Drawing for the job (mm, zero at the part's lowest x, y, z). Give positions to 0.01 mm unless a question says otherwise; leave off trailing zeros. Loops run counter-clockwise (first coordinate to the right, second up) from the corner with the lowest first, then second, coordinate; pieces in that order, holes last. Notation, with made-up numbers: (80, 7.25) -> (129, 7.25) arc R21 cw to (129, 35.25) -> close; hole circle Ø7 at (33, -1.75). An arc over 180 degrees is marked (long way). Answer in a Markdown table with one row per item. Add a question column.
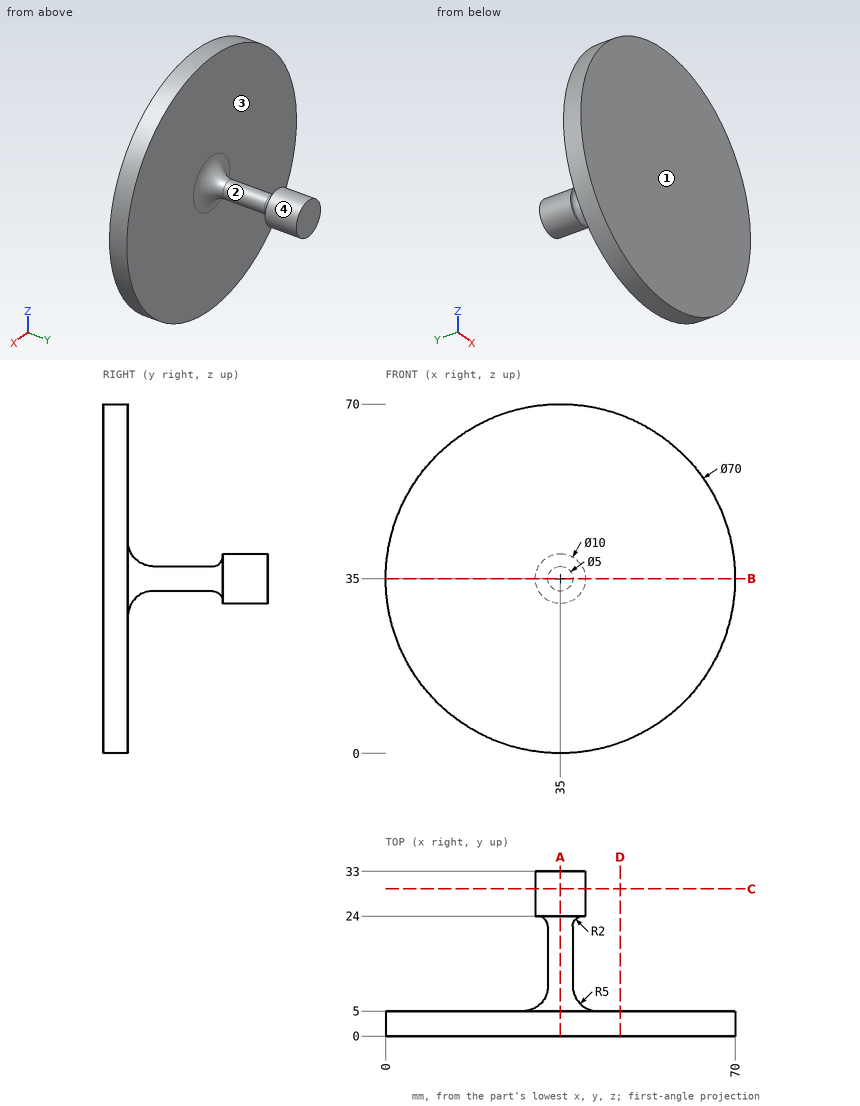
(1) Flat gauge pins, fed straight in: pin 1 Ø5 at (x, z) = (36.5, 33) entering from -Y; pin 2 Ø4 at (x, y) = (27.5, 22) entering from +Z; pin 3 Ø4 at (x, z) = (13.5, 32) entering from +Y; pin 4 Ø10 at (x, y) = (28, 8.5) entering from -Z. Where does each tip first touch, or does it go through?
(2) Wall check: line 1 along Y through (x, z) = (51, 53.5); line 2 along Y through (x, z) = (36, 30); line 3 along X through (y, z) = (3.5, 28). Give the ranges that are in metal, low to high. Write a range as from..to.
(3) Saw through at B-B, the plane z = 35. List the corners of the cut face in (x, y).
(4) Saw through at C-C, the plane y = 29.5. List the corners of the cut face in (x, z).
(5) Two-plate mould, pull along Y, no slides. Class the marked faces 1, 2, 3 and 4: released by +Y, released by -Y, zero draft, split by the parting line, or undercut.
(6) Saw through at D-D, the plane x = 47. List the corners of the cut face in (y, z), then the cut area to 3 significant figures.
(7) Saw through at A-A, the plane x = 35. List the corners of the cut face in (y, z), then the cut area to 3 significant figures.
Worked answers:
| question | item | result |
|---|---|---|
| 1 | pin 1 | y = 0 |
| 1 | pin 2 | through |
| 1 | pin 3 | y = 5 |
| 1 | pin 4 | z = 0.17 |
| 2 | line 1 | 0..5 |
| 2 | line 2 | 0..5.61 |
| 2 | line 3 | 0.71..69.29 |
| 3 | outline | (0, 0) -> (70, 0) -> (70, 5) -> (42.5, 5) arc R5 cw to (37.5, 10) -> (37.5, 22) arc R2 cw to (39.5, 24) -> (40, 24) -> (40, 33) -> (30, 33) -> (30, 24) -> (30.5, 24) arc R2 cw to (32.5, 22) -> (32.5, 10) arc R5 cw to (27.5, 5) -> (0, 5) -> close |
| 4 | outline | circle Ø10 at (35, 35) |
| 5 | face 1 | released by -Y |
| 5 | face 2 | undercut |
| 5 | face 3 | released by +Y |
| 5 | face 4 | zero draft |
| 6 | outline | (0, 2.12) -> (5, 2.12) -> (5, 67.88) -> (0, 67.88) -> close |
| 6 | area | 329 mm^2 |
| 7 | outline | (0, 0) -> (5, 0) -> (5, 27.5) arc R5 cw to (10, 32.5) -> (22, 32.5) arc R2 cw to (24, 30.5) -> (24, 30) -> (33, 30) -> (33, 40) -> (24, 40) -> (24, 39.5) arc R2 cw to (22, 37.5) -> (10, 37.5) arc R5 cw to (5, 42.5) -> (5, 70) -> (0, 70) -> close |
| 7 | area | 547 mm^2 |
